from build123d import *

# Parameters (mm, degrees)
SKETCH1_W           = 67
SKETCH1_H           = 75
BOSS_EXTRUDE1_DEPTH = 3
SKETCH2_R           = 1.5
CUT_EXTRUDE1_DEPTH  = 3
SKETCH3_R           = 3
SKETCH3_R_2         = 1
BOSS_EXTRUDE2_DEPTH = 3


with BuildPart() as part:
    # Sketch1 → Boss-Extrude1 (new body)
    with BuildSketch(Plane.XY):
        Rectangle(SKETCH1_W, SKETCH1_H)
    extrude(amount=BOSS_EXTRUDE1_DEPTH)

    # Sketch2 → Cut-Extrude1 (cut)
    with BuildSketch(Plane.XY.offset(3)):
        with Locations((-31, 35)):
            Circle(SKETCH2_R)
        with Locations((31, 35)):
            Circle(SKETCH2_R)
        with Locations((31, -35)):
            Circle(SKETCH2_R)
        with Locations((-31, -35)):
            Circle(SKETCH2_R)
    extrude(amount=-CUT_EXTRUDE1_DEPTH, mode=Mode.SUBTRACT)

    # Sketch3 → Boss-Extrude2 (add)
    # profile 1 of 2: a face of its own
    with BuildSketch(Plane.XY.offset(3)):
        with Locations(Location((-17.899535592, -13.876081532, 0), (0, 0, 180))):
            Circle(SKETCH3_R)
        with Locations((-17.899535592, -13.876081532)):
            Circle(SKETCH3_R_2, mode=Mode.SUBTRACT)
    # profile 2 of 2: a face of its own
    with BuildSketch(Plane.XY.offset(3)):
        with Locations(Location((19.600464408, -13.876081532, 0), (0, 0, 180))):
            Circle(SKETCH3_R)
        with Locations((19.600464408, -13.876081532)):
            Circle(SKETCH3_R_2, mode=Mode.SUBTRACT)
    extrude(amount=BOSS_EXTRUDE2_DEPTH)


solid = part.part
Design review of the part built by this model. Coordinates are the model's own, in mm. A direction names the side the tool comes from. Coordinates: 2 decimals unless noted, no trailing zeros. Loops run counter-clockwise (first coordinate to the right, second up) from the corner with the lowest first, then second, coordinate; pieces in that order, holes last.
Item 1: Add section A-A (x = -31). Write out the cut boundary in (y, z).
Completed:
outline: (-37.5, 0) - (-36.5, 0) - (-36.5, 3) - (-37.5, 3) - close; (-33.5, 0) - (33.5, 0) - (33.5, 3) - (-33.5, 3) - close; (36.5, 0) - (37.5, 0) - (37.5, 3) - (36.5, 3) - close
Item 2: Clearance check with flat-ended pins moving along their axes: pin 1 (2 mm diameter, centred on y = -13.5, z = 5, fed in from +X); pin 2 (5 mm diameter, centred on x = -31, y = 35, fed in from +Z); pin 3 (1 mm diameter, centred on x = 17.5, z = 5, fed in from -Y). State where each tip first meets the part, or that it passes through.
Completed:
pin 1: stops at x = 22.6
pin 2: stops at z = 3
pin 3: stops at y = -16.41
Item 3: Add section D-D (y = -27.5). Write out the cut boundary in (x, z).
Completed:
outline: (-33.5, 0) - (33.5, 0) - (33.5, 3) - (-33.5, 3) - close
Item 4: Wall thickness on L1, parallel to Y at x = -31, z = 1.8; L2, parallel to Z at x = -25.5, y = 7.5; L3, parallel to Y at x = 18.5, z = 5.05: over which ranges is each line inside the solid? List them lowest first.
Completed:
L1: y = -37.5 to -36.5, -33.5 to 33.5, 36.5 to 37.5
L2: z = 0 to 3
L3: y = -16.67 to -11.09
Item 5: Add section C-C (x = -20). Write out the cut boundary in (y, z), and give its area (3 significant figures).
Completed:
outline: (-37.5, 0) - (37.5, 0) - (37.5, 3) - (-11.73, 3) - (-11.73, 6) - (-16.02, 6) - (-16.02, 3) - (-37.5, 3) - close
area: 238 mm2
Item 6: For faces 4 (the cylindrical face through (-32.2, -35.9, 1.5)), 5 (the cylindrical face through (-16.976, -14.259, 4.479)), list the 3-axis set-ups (+Z, -Z, +X, -X, +Y, -Y) from which the entire face can be reached by the end or side of a thin tool; tool diameter is ignored.
Completed:
face 4: +Z, -Z
face 5: +Z
Item 7: Draft analysis for pull direction Y (two halves, no side actions). For faces 1 (the cylindrical face through (-32.2, 34.1, 1.5)), 2 (the flat face through (33.5, -1, 1)), 3 (the cylindrical face through (17.988, -16.406, 4.479)), state which applies: pulls with the +Y half, pulls with the -Y half, needs draft (parallel to the pull), parting line crosses it, or undercut.
Completed:
face 1: undercut
face 2: needs draft
face 3: parting line crosses it
Item 8: Add section B-B (y = 35). Write out the cut boundary in (x, z).
Completed:
outline: (-33.5, 0) - (-32.5, 0) - (-32.5, 3) - (-33.5, 3) - close; (-29.5, 0) - (29.5, 0) - (29.5, 3) - (-29.5, 3) - close; (32.5, 0) - (33.5, 0) - (33.5, 3) - (32.5, 3) - close
